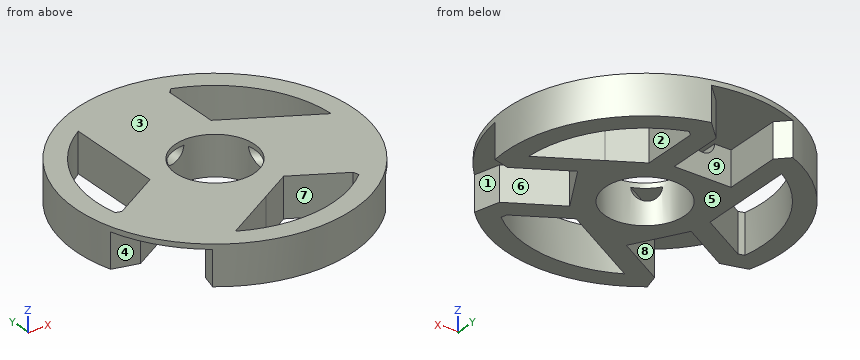
```python
from build123d import *

# Parameters (mm, degrees)
SKETCH1_R               = 250
BOSS_EXTRUDE1_DEPTH     = 5
SKETCH2_R               = 250
SKETCH2_W               = 57.5
SKETCH2_H               = 57.5
BOSS_EXTRUDE2_DEPTH     = 35
SKETCH3_R               = 250
SKETCH3_R_2             = 140
CUT_EXTRUDE1_DEPTH      = 356.808937493
CUT_EXTRUDE2_DEPTH      = 35
SKETCH5_R               = 40
CUT_EXTRUDE3_DEPTH      = 202.990098767
CUT_EXTRUDE4_REACH      = 261.517
CUT_EXTRUDE4_END_RADIUS = 40
CUT_EXTRUDE5_REACH      = 249.386
CUT_EXTRUDE5_END_RADIUS = 40
CUT_EXTRUDE6_REACH      = 261.517
CUT_EXTRUDE6_END_RADIUS = 40
CUT_EXTRUDE7_DEPTH      = 202.990098787


with BuildPart() as part:
    # Sketch1 → Boss-Extrude1 (new body)
    with BuildSketch(Plane.XY):
        Circle(SKETCH1_R)
    extrude(amount=-BOSS_EXTRUDE1_DEPTH)

    # Sketch2 → Boss-Extrude2 (add)
    with BuildSketch(Plane(origin=(0, 0, -5), x_dir=(-1, 0, 0), z_dir=(0, 0, -1))):
        with Locations(Location((0, 0, 0), (0, 0, 180))):
            Circle(SKETCH2_R)
        Polygon((-73.336524227, 7.022586012), (-123.132984945, -21.727413988), (-94.382984945, -71.523874706), (-44.586524227, -42.773874706), align=None, mode=Mode.SUBTRACT)
        with Locations((14, 88.75)):
            Rectangle(SKETCH2_W, SKETCH2_H, mode=Mode.SUBTRACT)
        Polygon((80.382984945, -95.772586012), (30.586524227, -67.022586012), (59.336524227, -17.226125294), (109.132984945, -45.976125294), align=None, mode=Mode.SUBTRACT)
    extrude(amount=BOSS_EXTRUDE2_DEPTH)

    # Sketch3 → Cut-Extrude1 (cut, through all)
    with BuildSketch(Plane(origin=(0, 0, -40), x_dir=(-1, 0, 0), z_dir=(0, 0, -1))):
        Circle(SKETCH3_R)
        Circle(SKETCH3_R_2, mode=Mode.SUBTRACT)
    extrude(amount=-CUT_EXTRUDE1_DEPTH, mode=Mode.SUBTRACT)

    # Sketch4 → Cut-Extrude2 (cut)
    with BuildSketch(Plane(origin=(0, 0, -40), x_dir=(-1, 0, 0), z_dir=(0, 0, -1))):
        with BuildLine():
            Line((42.75, 117.5), (54.293475361, 129.043475361))
            ThreePointArc((54.293475361, 129.043475361), (11.083221394, 139.560604053), (-33.245383921, 135.995383921))
            Line((-33.245383921, 135.995383921), (-14.75, 117.5))
            Line((-14.75, 117.5), (42.75, 117.5))
        make_face()
        with BuildLine():
            Line((-123.132984945, -21.727413988), (-138.901665536, -17.502208758))
            ThreePointArc((-138.901665536, -17.502208758), (-126.404639174, -60.181950743), (-101.152765313, -96.789038995))
            Line((-101.152765313, -96.789038995), (-94.382984945, -71.523874706))
            Line((-94.382984945, -71.523874706), (-123.132984945, -21.727413988))
        make_face()
        with BuildLine():
            Line((80.382984945, -95.772586012), (84.608190175, -111.541266603))
            ThreePointArc((84.608190175, -111.541266603), (115.32141778, -79.378653309), (134.398149234, -39.206344926))
            Line((134.398149234, -39.206344926), (109.132984945, -45.976125294))
            Line((109.132984945, -45.976125294), (80.382984945, -95.772586012))
        make_face()
    extrude(amount=-CUT_EXTRUDE2_DEPTH, mode=Mode.SUBTRACT)

    # Sketch5 → Cut-Extrude3 (cut, through all)
    with BuildSketch(Plane(origin=(0, 0, -40), x_dir=(-1, 0, 0), z_dir=(0, 0, -1))):
        Circle(SKETCH5_R)
    extrude(amount=-CUT_EXTRUDE3_DEPTH, mode=Mode.SUBTRACT)

    # Cut-Extrude4: up to this cylinder (the profile starts outside it)
    cut_extrude4_end = Plane(origin=(0, 0, -10.092958), z_dir=(0, 0, -1)) * Cylinder(CUT_EXTRUDE4_END_RADIUS, 604.034, mode=Mode.PRIVATE)
    # Sketch7 → Cut-Extrude4 (cut, up to the surface)
    with BuildSketch(Plane(origin=(-51.961524227, -30, 0), x_dir=(0, 0, 1), z_dir=(-0.866025403784445, -0.49999999999998906, 0)), mode=Mode.PRIVATE) as cut_extrude4_sk1:
        with BuildLine():
            Line((-5, -26), (-5, -2))
            ThreePointArc((-5, -2), (-17, -14), (-5, -26))
        make_face()
    cut_extrude4_tool1 = extrude(cut_extrude4_sk1.sketch, amount=-CUT_EXTRUDE4_REACH, mode=Mode.PRIVATE) - cut_extrude4_end
    add(cut_extrude4_tool1.solids().sort_by_distance((-44.961524, -42.124356, -10.092958))[0], mode=Mode.SUBTRACT)

    # Cut-Extrude5: up to this cylinder (the profile starts outside it)
    cut_extrude5_end = Plane(origin=(0, 0, -10.092958), z_dir=(0, 0, -1)) * Cylinder(CUT_EXTRUDE5_END_RADIUS, 579.772, mode=Mode.PRIVATE)
    # Sketch8 → Cut-Extrude5 (cut, up to the surface)
    with BuildSketch(Plane(origin=(0, 60, 0), x_dir=(1, 0, 0), z_dir=(0, 1, 0)), mode=Mode.PRIVATE) as cut_extrude5_sk1:
        with BuildLine():
            Line((-26, 5), (-2, 5))
            ThreePointArc((-2, 5), (-14, 17), (-26, 5))
        make_face()
    cut_extrude5_tool1 = extrude(cut_extrude5_sk1.sketch, amount=-CUT_EXTRUDE5_REACH, mode=Mode.PRIVATE) - cut_extrude5_end
    add(cut_extrude5_tool1.solids().sort_by_distance((-14, 60, -10.092958))[0], mode=Mode.SUBTRACT)

    # Cut-Extrude6: up to this cylinder (the profile starts outside it)
    cut_extrude6_end = Plane(origin=(0, 0, -10.092958), z_dir=(0, 0, -1)) * Cylinder(CUT_EXTRUDE6_END_RADIUS, 604.034, mode=Mode.PRIVATE)
    # Sketch9 → Cut-Extrude6 (cut, up to the surface)
    with BuildSketch(Plane(origin=(51.961524227, -30, 0), x_dir=(0, 0, -1), z_dir=(0.8660254037844376, -0.5000000000000019, 0)), mode=Mode.PRIVATE) as cut_extrude6_sk1:
        with BuildLine():
            Line((5, 26), (5, 2))
            ThreePointArc((5, 2), (17, 14), (5, 26))
        make_face()
    cut_extrude6_tool1 = extrude(cut_extrude6_sk1.sketch, amount=-CUT_EXTRUDE6_REACH, mode=Mode.PRIVATE) - cut_extrude6_end
    add(cut_extrude6_tool1.solids().sort_by_distance((58.961524, -17.875644, -10.092958))[0], mode=Mode.SUBTRACT)

    # Sketch10 → Cut-Extrude7 (cut, through all)
    with BuildSketch(Plane(origin=(0, 0, -40), x_dir=(-1, 0, 0), z_dir=(0, 0, -1))):
        with BuildLine():
            Line((62.75, 40), (62.75, 3.897114317))
            Line((62.75, 3.897114317), (111.958595593, -24.513481595))
            Line((111.958595593, -24.513481595), (117.784487806, -22.952438481))
            ThreePointArc((117.784487806, -22.952438481), (109.860573104, 48.276852396), (62.75, 102.286057212))
            Line((62.75, 102.286057212), (62.75, 40))
        make_face()
        with BuildLine():
            Line((3.266016151, -74.343094087), (-28, -56.291651246))
            Line((-28, -56.291651246), (-77.208595593, -84.702247158))
            Line((-77.208595593, -84.702247158), (-78.769638706, -90.528139372))
            ThreePointArc((-78.769638706, -90.528139372), (-13.121305962, -119.28047338), (57.207323999, -105.486122694))
            Line((57.207323999, -105.486122694), (3.266016151, -74.343094087))
        make_face()
        with BuildLine():
            Line((-66.016016151, 34.343094087), (-34.75, 52.394536929))
            Line((-34.75, 52.394536929), (-34.75, 109.215728753))
            Line((-34.75, 109.215728753), (-39.0148491, 113.480577852))
            ThreePointArc((-39.0148491, 113.480577852), (-96.739267142, 71.003620984), (-119.957323999, 3.200065481))
            Line((-119.957323999, 3.200065481), (-66.016016151, 34.343094087))
        make_face()
    extrude(amount=-CUT_EXTRUDE7_DEPTH, mode=Mode.SUBTRACT)


solid = part.part
```
Geometry check sheet. Reference: the model listing, model coordinates, mm. Face numbers are marked on the shaded views. A direction names the side the tool comes from. Give positions to 0.01 mm unless a question says otherwise; leave off trailing zeros. Loops run counter-clockwise (first coordinate to the right, second up) from the corner with the lowest first, then second, coordinate; pieces in that order, holes last. Notation, with made-up numbers: (25, 72) - (69, 72) arc R7 cw to (69, 77) - close; hole circle Ø2 at (28, 59.25). An arc over 180 degrees is marked (long way). Use CSV: the item, a comma, the result in double quotes. Start each with the question number.
Q1. Section check B-B, the plane y = 84.5. Record the cut outline in (x, z).
Q2. Release check for a two-part mould opening along X. For the marked faces 1, 2, 3 and 4 record: +X half, -X half, draft (parallel to the pull), parting line (faces both ways), or undercut.
Q3. Section check C-C, the plane x = -100. Record the cut outline in (y, z), and give its area (3 significant figures).
Q4. Go/stop test with flat-tipped pins: pin 1 Ø5 at (y, z) = (30.5, -17) entering from -X; pin 2 Ø6 at (x, z) = (55, -30.5) entering from +Y; pin 3 Ø2 at (y, z) = (-20, -4) entering from -X. Record where each tip stops, or that it passes through.
Q5. Section check A-A, the plane z = -33. Count the separate pieces of the cut face and the enclosed holes in it, and give its area (3 significant figures).
Q6. Section check D-D, the plane x = 23. Record the cut outline in (y, z).
Q7. Scan lines: probe 1 along X at (y, z) = (0, -11); probe 2 along X at (y, z) = (77, -34); probe 3 along Y at (x, z) = (0, -18.5). Record each from-to range of solid material in increasing order. Write a range as from..to.
Q8. Access from +Z, -Z, +X, -X, +Y, -Y to the whole of each face (thin tool, end or side, straight path). Record for the marked faces 5, 6, 7, 8 and 9.
Findings below:
1,outline,"(-111.62, -40) - (-85.2, -40) - (-85.2, 0) - (-111.62, 0) - close; (-62.75, -40) - (-42.75, -40) - (-42.75, -5) - (14.75, -5) - (14.75, -40) - (34.75, -40) - (34.75, 0) - (-62.75, 0) - close; (85.2, -40) - (111.62, -40) - (111.62, 0) - (85.2, 0) - close"
2,face 1,"+X half"
2,face 2,"undercut"
2,face 3,"draft"
2,face 4,"-X half"
3,outline,"(-97.98, -5) - (-40.7, -5) - (-40.7, -40) - (-17.61, -40) - (-17.61, 0) - (-97.98, 0) - close; (66.33, -40) - (97.98, -40) - (97.98, 0) - (66.33, 0) - close"
3,area,"2,480 mm^2"
4,pin 1,"stops at x = -137.17"
4,pin 2,"stops at y = 129.98"
4,pin 3,"stops at x = -138.7"
5,separate pieces,"1"
5,enclosed holes,"4"
5,area,"27,700 mm^2"
6,outline,"(-138.1, -40) - (-117.78, -40) - (-117.78, 0) - (-138.1, 0) - close; (-59.18, -40) - (-32.73, -40) - (-32.73, 0) - (-59.18, 0) - close; (32.73, -40) - (125.75, -40) - (125.75, -5) - (138.1, -5) - (138.1, 0) - (32.73, 0) - close"
7,probe 1,"x = -140..-120, -69.5..-40, 48.78..69.28, 85.5..140"
7,probe 2,"x = -116.92..-92.04, -62.75..-42.75, 14.75..34.75, 92.04..116.92"
7,probe 3,"y = -140..-120, -72.46..-40, 40..60"
8,face 5,"-Z, +X, -X, +Y, -Y"
8,face 6,"-Z, +X"
8,face 7,"+Z, -Z"
8,face 8,"-Z, -X"
8,face 9,"-Z, +Y"
